Can you work these out from the model? Positions are in its coordinate system, mm. A direction names the side the tool comes from. Coordinates: 2 decimals unless noted, no trailing zeros. Order: outer loops, then holes, each group sorted by start corner. A loop starts at its lowest first (then second) coordinate and runs counter-clockwise, first axis right, second up. Notation, with made-up numbers: M 86.5,65.5 L 138.5,65.5 A30 ccw 138.5,98.5 Z; hole C 22,8.5 d10. An arc over 180 degrees is marked long. Answer as a JSON object with one key per item and string values.
from build123d import *

# Parameters (mm, degrees)
F1_DEPTH  = 28
F2_W      = 211.909
F2_H      = 3
F3_DEPTH  = 15
F4_W      = 70
F4_H      = 3
F5_DEPTH  = 15
F7_DEPTH  = 3
F8_R      = 18.2181512029
F10_DEPTH = 3
F11_R     = 18.218


with BuildPart() as f1:
    # F0 (on Top) → F1 (new body)
    with BuildSketch(Plane.XY):
        with BuildLine():
            Line((23.2926856095, 0), (-81.7073143905, 0))
            Line((-81.7073143905, 0), (-81.7073143905, -15))
            Line((-81.7073143905, -15), (130.2926856095, -15))
            Line((130.2926856095, -15), (130.2926856095, 17))
            Line((130.2926856095, 17), (60.2926856095, 17))
            add(Edge.make_bspline(
                [(60.2926856095, 17), (47.0403235396, 17), (38.2657825675, 0), (23.2926856095, 0)],
                knots=[0, 0, 0, 0, 40.718546143, 40.718546143, 40.718546143, 40.718546143], degree=3))
        make_face()
    extrude(amount=-F1_DEPTH)

    # F2 (on face) → F3 (join)
    with BuildSketch(Plane(origin=(0, 0, 0), x_dir=(-1, 0, 0), z_dir=(0, 1, 0))):
        with Locations((-24.2471856095, -1.5)):
            Rectangle(F2_W, F2_H)
        with Locations((-24.2471856095, -26.5)):
            Rectangle(F2_W, F2_H)
    extrude(amount=F3_DEPTH)

    # F4 (on face) → F5 (join)
    with BuildSketch(Plane(origin=(0, 17, 0), x_dir=(-1, 0, 0), z_dir=(0, 1, 0))):
        with Locations((-95.2926856095, -26.5)):
            Rectangle(F4_W, F4_H)
        with Locations((-95.2926856095, -1.5)):
            Rectangle(F4_W, F4_H)
    extrude(amount=F5_DEPTH)

    # F6 (on face) → F7 (join)
    with BuildSketch(Plane.XY):
        Polygon((64.7905170918, 0), (60.2926856095, 32), (21.7418372631, 15), (26.0446537286, -15), align=None)
    extrude(amount=-F7_DEPTH)

    # F8
    f8_edges = [f1.edges().sort_by_distance(p)[0] for p in [
        (60.292686, 32, -1.5),
        (21.741837, 15, -1.5),
    ]]
    fillet(f8_edges, radius=F8_R)

    # F9 (on face) → F10 (join)
    with BuildSketch(Plane(origin=(0, 0, -28), x_dir=(1, 0, 0), z_dir=(0, 0, -1))):
        Polygon((24.2926856095, -15), (60.2926856095, -32), (60.2926856095, -17), (52.3001670697, -15), align=None)
    extrude(amount=-F10_DEPTH)

    # F11
    f11_edges = [f1.edges().sort_by_distance(p)[0] for p in [
        (60.292686, 32, -26.5),
        (24.292686, 15, -26.5),
    ]]
    fillet(f11_edges, radius=F11_R)


solid = f1.part
Item 1: I want a section at C-C, the plane x = 80. Write out the boundary of the cut face in (y, z), plus the area to 3 significant figures.
Answers follow:
{"outline": "M -15,-28 L 32,-28 L 32,-25 L 17,-25 L 17,-3 L 32,-3 L 32,0 L -15,0 Z", "area": "986 mm^2"}
Item 2: I want a section at B-B, the plane y = 27.5. Write out the boundary of the cut face in (x, z), plus the area to 3 significant figures.
Answers follow:
{"outline": "M 50.09,-3 L 130.29,-3 L 130.29,0 L 50.09,0 Z; M 50.76,-28 L 130.29,-28 L 130.29,-25 L 50.76,-25 Z", "area": "479 mm^2"}
Item 3: Please list where these lines run through material, in increasing order: line 1 (Z direction, x = -46, y = 9.5); line 2 (Y direction, x = 62, z = -19.5); line 3 (Y direction, x = -26, z = -10.75).
Answers follow:
{"line 1": "z = -28 to -25, -3 to 0", "line 2": "y = -15 to 17", "line 3": "y = -15 to 0"}
Item 4: I'm going to push flat-ended pins straight in: pin 1 (1.5 mm diameter, centred on x = -13, z = -27, fed in from +Y); pin 2 (4 mm diameter, centred on x = 47.5, z = -18, fed in from +Y); pin 3 (1.5 mm diameter, centred on y = 19.5, z = -5, fed in from -X). Where does each tip first touch, or does it pass through?
Answers follow:
{"pin 1": "stops at y = 15", "pin 2": "stops at y = 13.46", "pin 3": "passes through"}
Item 5: I want a section at A-A, the plane x = -13. Write out the boundary of the cut face in (y, z), plus the area to 3 significant figures.
Answers follow:
{"outline": "M -15,-28 L 15,-28 L 15,-25 L 0,-25 L 0,-3 L 15,-3 L 15,0 L -15,0 Z", "area": "510 mm^2"}
Item 6: Which directions (+Z, -Z, +X, -X, +Y, -Y) give clear straight access to the entire face, cutting with the end or side of a thin tool? Please do faces 4 (the flat face through (-28, 0, -14)), 5 (the flat face through (96, 17, -14)), 6 (the flat face through (42.092, 23.405, -26.521)).
Answers follow:
{"face 4": "-X, +Y", "face 5": "+X, -X, +Y", "face 6": "-Z, -X, +Y"}
Item 7: If we mould it in two halves opening along Z, with no side actions, what happens to faces 1 (the flat face through (41.24, 23.6, -1.48)), 2 (the flat face through (23, 3, -28)), 3 (the flat face through (26, 16, -3))? For each: pulls with the +Z half, pulls with the -Z half, needs draft (parallel to the pull), parting line crosses it, or undercut.
Answers follow:
{"face 1": "needs draft", "face 2": "pulls with the -Z half", "face 3": "undercut"}
